```python
from build123d import *

# Parameters (mm, degrees)
SKETCH2_R             = 57.15
BOSS_EXTRUDE1_DEPTH   = 2.54
SKETCH3_R             = 5.08
BOSS_EXTRUDE2_DEPTH   = 12.7
CIRPATTERN1_COUNT     = 4
F_8_32_TAPPED_HOLE1_D = 3.4544
CIRPATTERN2_COUNT     = 4


with BuildPart() as part:
    # Sketch2 → Boss-Extrude1 (new body)
    with BuildSketch(Plane(origin=(0, 0, 0), x_dir=(1, 0, 0), z_dir=(0, 1, 0))):
        with Locations(Location((0, 0, 0), (0, 0, 270))):
            Circle(SKETCH2_R)
    extrude(amount=BOSS_EXTRUDE1_DEPTH)

    # Sketch3 → Boss-Extrude2 (add)
    with BuildSketch(Plane.XZ):
        with Locations(Location((-32.710383859, -28.187642467, 0), (0, 0, 90))):
            Circle(SKETCH3_R)
    boss_extrude2 = extrude(amount=BOSS_EXTRUDE2_DEPTH)

    # CirPattern1: Boss-Extrude2 ×4 about axis
    cirpattern1_axis = Axis((0, 0, 0), (0, 1, 0))
    for i in range(1, CIRPATTERN1_COUNT):
        add(boss_extrude2.rotate(cirpattern1_axis, i * 360 / CIRPATTERN1_COUNT))

    # #8-32 Tapped Hole1 (through all)
    with Locations(Plane(origin=(0, 2.54, 0), x_dir=(1, 0, 0), z_dir=(0, 1, 0))):
        with Locations((-53.34, 0)):
            f_8_32_tapped_hole1 = Hole(F_8_32_TAPPED_HOLE1_D / 2)

    # CirPattern2: #8-32 Tapped Hole1 ×4 about axis
    cirpattern2_axis = Axis((0, 0, 0), (0, 1, 0))
    for i in range(1, CIRPATTERN2_COUNT):
        add(f_8_32_tapped_hole1.rotate(cirpattern2_axis, i * 360 / CIRPATTERN2_COUNT), mode=Mode.SUBTRACT)


solid = part.part
```
Part model, mm, in its own coordinate system. A direction names the side the tool comes from. Give positions to 0.01 mm unless a question says otherwise; leave off trailing zeros. Order: outer loops, then holes, each group sorted by start corner. A loop starts at its lowest first (then second) coordinate and runs counter-clockwise, first axis right, second up. Notation, with made-up numbers: (-24, 59) - (-6, 59) arc R30 cw to (-6, 85) - close; hole circle Ø10 at (82.5, 49). An arc over 180 degrees is marked (long way). Use one line per item in the form item = value.
Item 1: Slice it at A-A on z = 0. Give the cut face in (x, y), and give its area (3 significant figures).
Solution:
outline = (-57.15, 0) - (-55.07, 0) - (-55.07, 2.54) - (-57.15, 2.54) - close; (-51.61, 0) - (51.61, 0) - (51.61, 2.54) - (-51.61, 2.54) - close; (55.07, 0) - (57.15, 0) - (57.15, 2.54) - (55.07, 2.54) - close
area = 273 mm2
Item 2: Which spindle directions (+Z, -Z, +X, -X, +Y, -Y) get a long thin tool onto all of the face, cutting with end or side? Do faces 4 (the face through (-23.342, -6.261, 34.236)), 5 (the face through (33, -12.7, 28)). Say none if no direction does.
Solution:
face_4 = -Y
face_5 = +Z, -Z, +X, -X, -Y
Item 3: Slice it at B-B on x = 0. Give the cut face in (y, z).
Solution:
outline = (0, -57.15) - (2.54, -57.15) - (2.54, -55.07) - (0, -55.07) - close; (0, -51.61) - (2.54, -51.61) - (2.54, 51.61) - (0, 51.61) - close; (0, 55.07) - (2.54, 55.07) - (2.54, 57.15) - (0, 57.15) - close
Item 4: Two-plate mould, pull along X, no slides. Class faces 1 (the face through (-51.614, 1.252, -0.076)), 2 (the face through (1, 2.54, -1)), 3 (the face through (2.513, 1.252, -57.095)): released by +X, released by -X, zero draft, split by the parting line, or undercut.
Solution:
face_1 = undercut
face_2 = zero draft
face_3 = split by the parting line
Item 5: Pin check, flat tips, straight feed: pin 1 Ø3 at (x, z) = (0, 53.34) entering from +Y; pin 2 Ø8 at (x, y) = (27, -6) entering from -Z; pin 3 Ø4 at (x, z) = (-53.34, 0) entering from -Y; pin 4 Ø6 at (x, y) = (-33, -10) entering from +Z. Stop position of each tip, or through.
Solution:
pin_1 = through
pin_2 = -37.79
pin_3 = 0
pin_4 = 37.46
Item 6: Slice it at D-D on y = -4.5. Give the cut face in (x, z).
Solution:
outline = circle Ø10.16 at (-32.71, -28.19); circle Ø10.16 at (-28.19, 32.71); circle Ø10.16 at (28.19, -32.71); circle Ø10.16 at (32.71, 28.19)
Item 7: Probe probe 1 along Y at (x, z) = (-4, 20); probe 2 along Z at (x, y) = (-30.5, -1); probe 3 along X at (y, z) = (-6, -36). List the from-to ranges inside material, lowest first. Write a range as from..to.
Solution:
probe_1 = 0..2.54
probe_2 = -32.76..-23.61, 28.19..37.23
probe_3 = 24.32..32.06
Item 8: Slice it at C-C on z = 53.34. Give the cut face in (x, y).
Solution:
outline = (-20.52, 0) - (-1.73, 0) - (-1.73, 2.54) - (-20.52, 2.54) - close; (1.73, 0) - (20.52, 0) - (20.52, 2.54) - (1.73, 2.54) - close
